```python
from build123d import *

# Parameters (mm, degrees)
SKETCH085_R  = 1.5
PAD064_DEPTH = 25
SKETCH082_R  = 1.5
PAD063_DEPTH = 25


with BuildPart() as pad064:
    # Sketch085 → Pad064 (new body, symmetric)
    with BuildSketch(Plane.XY):
        with Locations((-12.5, 0)):
            Circle(SKETCH085_R)
    extrude(amount=PAD064_DEPTH, both=True)


with BuildPart() as screwcutout:
    # Sketch082 → Pad063 (new body, symmetric)
    with BuildSketch(Plane.XZ):
        with Locations((-12.5, 0)):
            Circle(SKETCH082_R)
    extrude(amount=PAD063_DEPTH, both=True)

    # Fusion004024: union Pad064
    add(pad064.part)


with BuildPart() as endcap:
    # Sketch083 → Revolution (revolve)
    with BuildSketch(Plane.XY):
        Polygon((-15, 3), (-15, 12), (-9.5, 12), (-9.5, 10), (-11, 8), (-11, 4.25), (-14, 4.25), (-14, 3), align=None)
    revolve(axis=Axis((0, 0, 0), (1, 0, 0)))

    # Cut007019003: cut ScrewCutout
    add(screwcutout.part, mode=Mode.SUBTRACT)


solid = endcap.part
```
Check sheet for the modelled part. Datum: model origin and axes. Units: mm. A direction names the side the tool comes from. Round coordinates to 2 decimals unless told otherwise and drop trailing zeros. Loops run counter-clockwise (first coordinate to the right, second up) from the corner with the lowest first, then second, coordinate; pieces in that order, holes last. Notation, with made-up numbers: (21.5, 30.25) -> (40.5, 30.25) arc R33 cw to (40.5, 65.25) -> close; hole circle Ø7 at (75.25, 82.25). An arc over 180 degrees is marked (long way). Answer in a Markdown table with one row per item.
Q1. Go/stop test with flat-tipped pins: P1, Ø3, axis at y = -4, z = -6, coming from the +X side; P2, Ø1, axis at x = -11, z = -7.5, coming from the +Y side; P3, Ø2.5, axis at x = -12.5, y = 0, coming from the -Z side; P4, Ø4, axis at y = -0.5, z = 1, coming from the +X side. Record where each tip stops, or that it passes through.
Data:
| item | result |
|---|---|
| P1 | stops at x = -10.47 |
| P2 | stops at y = 9.75 |
| P3 | passes through |
| P4 | stops at x = -14 |
Q2. Release check for a two-part mould opening along Z. For faces 1 (the face through (-11, -4, -4)), 2 (the face through (-12.212, 11.446, 3.604)), 3 (the face through (-9.5, -5, 9)), 4 (the face through (-12.52, 3.04, 2.97)) record: released by +Z, released by -Z, zero draft, split by the parting line, or undercut.
Data:
| item | result |
|---|---|
| face 1 | undercut |
| face 2 | split by the parting line |
| face 3 | zero draft |
| face 4 | undercut |
Q3. Set-up check for faces 5 (the face through (-14, 1, 3)), 6 (the face through (-14.5, -3, 0.1)): record each of +Z, -Z, +X, -X, +Y, -Y from which the full face is reachable in a straight line by a thin tool's end or side.
Data:
| item | result |
|---|---|
| face 5 | +X |
| face 6 | +X, -X |
Q4. Sectioned sample at B-B on z = 0.75. Give the number of separate pieces and of enclosed holes in the cut face, then the cut area to 3 significant figures.
Data:
| item | result |
|---|---|
| separate pieces | 4 |
| enclosed holes | 0 |
| area | 33.4 mm^2 |
Q5. Thickness scan on L1, parallel to Z at x = -14.8, y = 0; L2, parallel to X at y = -3.75, z = -1; L3, parallel to X at y = 0, z = -9.25. Record the ranges inside material, lowest first.
Data:
| item | result |
|---|---|
| L1 | z = -12 to -3, 3 to 12 |
| L2 | x = -15 to -14 |
| L3 | x = -15 to -14, -11 to -10.06 |
Q6. Sectioned sample at A-A on x = -12.5. Enter the section's corners in (y, z), then the cut area to 3 significant figures.
Data:
| item | result |
|---|---|
| outline | (-11.91, -1.5) arc R12 ccw to (-1.5, -11.91) -> (-1.5, -3.98) arc R4.25 cw to (-3.98, -1.5) -> close; (-11.91, 1.5) -> (-3.98, 1.5) arc R4.25 cw to (-1.5, 3.98) -> (-1.5, 11.91) arc R12 ccw to start; (1.5, -11.91) arc R12 ccw to (11.91, -1.5) -> (3.98, -1.5) arc R4.25 cw to (1.5, -3.98) -> close; (1.5, 3.98) arc R4.25 cw to (3.98, 1.5) -> (11.91, 1.5) arc R12 ccw to (1.5, 11.91) -> close |
| area | 302 mm^2 |
